from build123d import *

# Parameters (mm, degrees)
SKETCH001_W      = 53
SKETCH001_H      = 17
SKETCH001_R      = 1.25
EXTRUDE002_DEPTH = 4.5
EXTRUDE001_DEPTH = 50
EXTRUDE_DEPTH    = 50
EXTRUDE003_DEPTH = 4.5


with BuildPart() as extrude002:
    # Sketch001 → Extrude002 (new body)
    with BuildSketch(Plane.XZ):
        with Locations((14.5, -8.5)):
            Rectangle(SKETCH001_W, SKETCH001_H)
        with Locations((-8.8, -3.75)):
            Circle(SKETCH001_R, mode=Mode.SUBTRACT)
        with Locations((-8.8, -13.25)):
            Circle(SKETCH001_R, mode=Mode.SUBTRACT)
        with Locations((37.8, -13.25)):
            Circle(SKETCH001_R, mode=Mode.SUBTRACT)
        with Locations((37.8, -3.75)):
            Circle(SKETCH001_R, mode=Mode.SUBTRACT)
    extrude(amount=EXTRUDE002_DEPTH)


with BuildPart() as extrude001:
    # Sketch → Extrude001 (new body)
    with BuildSketch(Plane.XZ):
        Polygon((0, 0), (29, 0), (29, 8), (29, 11.7), (29, 14.4), (21.25, 14.4), (21.25, 11.7), (24, 11.7), (24, 8), (5, 8), (5, 11.7), (7.75, 11.7), (7.75, 14.4), (0, 14.4), (0, 11.7), (0, 8), align=None)
    extrude(amount=EXTRUDE001_DEPTH)


with BuildPart() as extrude_body:
    # Sketch → Extrude (new body)
    with BuildSketch(Plane.XZ):
        Polygon((0, 0), (29, 0), (29, 8), (29, 11.7), (29, 14.4), (21.25, 14.4), (21.25, 11.7), (24, 11.7), (24, 8), (5, 8), (5, 11.7), (7.75, 11.7), (7.75, 14.4), (0, 14.4), (0, 11.7), (0, 8), align=None)
    extrude(amount=EXTRUDE_DEPTH)


with BuildPart() as fusion:
    # Sketch001 → Extrude003 (new body)
    with BuildSketch(Plane.XZ):
        with Locations((14.5, -8.5)):
            Rectangle(SKETCH001_W, SKETCH001_H)
        with Locations((-8.8, -3.75)):
            Circle(SKETCH001_R, mode=Mode.SUBTRACT)
        with Locations((-8.8, -13.25)):
            Circle(SKETCH001_R, mode=Mode.SUBTRACT)
        with Locations((37.8, -13.25)):
            Circle(SKETCH001_R, mode=Mode.SUBTRACT)
        with Locations((37.8, -3.75)):
            Circle(SKETCH001_R, mode=Mode.SUBTRACT)
    extrude(amount=EXTRUDE003_DEPTH)

    # Fusion: union Extrude002, Extrude001, Extrude body
    add(extrude002.part)
    add(extrude001.part)
    add(extrude_body.part)


solid = fusion.part
Verification items for the finished model (mm, model axes). A direction names the side the tool comes from. Coordinates: 2 decimals unless noted, no trailing zeros. Write each loop counter-clockwise with the first axis right and the second up, starting at its lowest first coordinate (ties: lowest second). Pieces come first, ordered by that corner, then holes. Notation, with made-up numbers: M 72,42.25 L 78,42.25 A26 cw 78,79.25 Z; hole C -22.5,-34.75 d2. An arc over 180 degrees is marked long. One line per question, with ' | ' between items.
1) Access from +Z, -Z, +X, -X, +Y, -Y to the whole of each face (thin tool, end or side, straight path). Record for faces 4 (the face through (-6, -2, 0)), 5 (the face through (21.25, -25, 13)), 6 (the face through (15, -25, 8)).
Solutions:
face 4: +Z, -X, +Y, -Y | face 5: +Z, +Y, -Y | face 6: +Y, -Y
2) Sectioned sample at C-C on x = -8.8. Record the cut outline in (y, z), then the cut area to 3 significant figures.
Solutions:
outline: M -4.5,-17 L 0,-17 L 0,-14.5 L -4.5,-14.5 Z; M -4.5,-12 L 0,-12 L 0,-5 L -4.5,-5 Z; M -4.5,-2.5 L 0,-2.5 L 0,0 L -4.5,0 Z | area: 54.0 mm^2
3) Release check for a two-part mould opening along X. For faces 1 (the face through (0, -25, 7)), 2 (the face through (4, -25, 14.4)), 3 (the face through (39, -2.2, -12.9)) record: +X half, -X half, draft (parallel to the pull), parting line (faces both ways), or undercut.
Solutions:
face 1: -X half | face 2: draft | face 3: undercut
4) Sectioned sample at B-B on z = -13.25. Record the cut outline in (x, y), then the cut area to 3 significant figures.
Solutions:
outline: M -12,-4.5 L -10.05,-4.5 L -10.05,0 L -12,0 Z; M -7.55,-4.5 L 36.55,-4.5 L 36.55,0 L -7.55,0 Z; M 39.05,-4.5 L 41,-4.5 L 41,0 L 39.05,0 Z | area: 216 mm^2
5) Material ranges on L1, parallel to Z at x = 37.8, y = -2.5; L2, parallel to Z at x = 37, y = -2; L3, parallel to X at y = -42, z = 10, recorded low to high.
Solutions:
L1: -17 to -14.5, -12 to -5, -2.5 to 0 | L2: -17 to -14.21, -12.29 to -4.71, -2.79 to 0 | L3: 0 to 5, 24 to 29
6) Sectioned sample at A-A on x = 7. Record the cut outline in (y, z).
Solutions:
outline: M -50,0 L -4.5,0 L -4.5,-17 L 0,-17 L 0,8 L -50,8 Z; M -50,11.7 L 0,11.7 L 0,14.4 L -50,14.4 Z
7) Depth check by flat-ended pin: pin 1 Ø5 at (x, y) = (33.5, -17.5) entering from -Z; pin 2 Ø7 at (y, z) = (-30.5, 6) entering from -X; pin 3 Ø5 at (x, y) = (37, -2.5) entering from +Z; pin 4 Ø8.5 at (x, z) = (6, -5) entering from -Y. Enter the tip coordinate at first touch or a pass-through.
Solutions:
pin 1: through | pin 2: x = 0 | pin 3: z = 0 | pin 4: y = -4.5
8) Sectioned sample at D-D on y = -35.5. Record the cut outline in (x, z), then the cut area to 3 significant figures.
Solutions:
outline: M 0,0 L 29,0 L 29,14.4 L 21.25,14.4 L 21.25,11.7 L 24,11.7 L 24,8 L 5,8 L 5,11.7 L 7.75,11.7 L 7.75,14.4 L 0,14.4 Z | area: 311 mm^2
